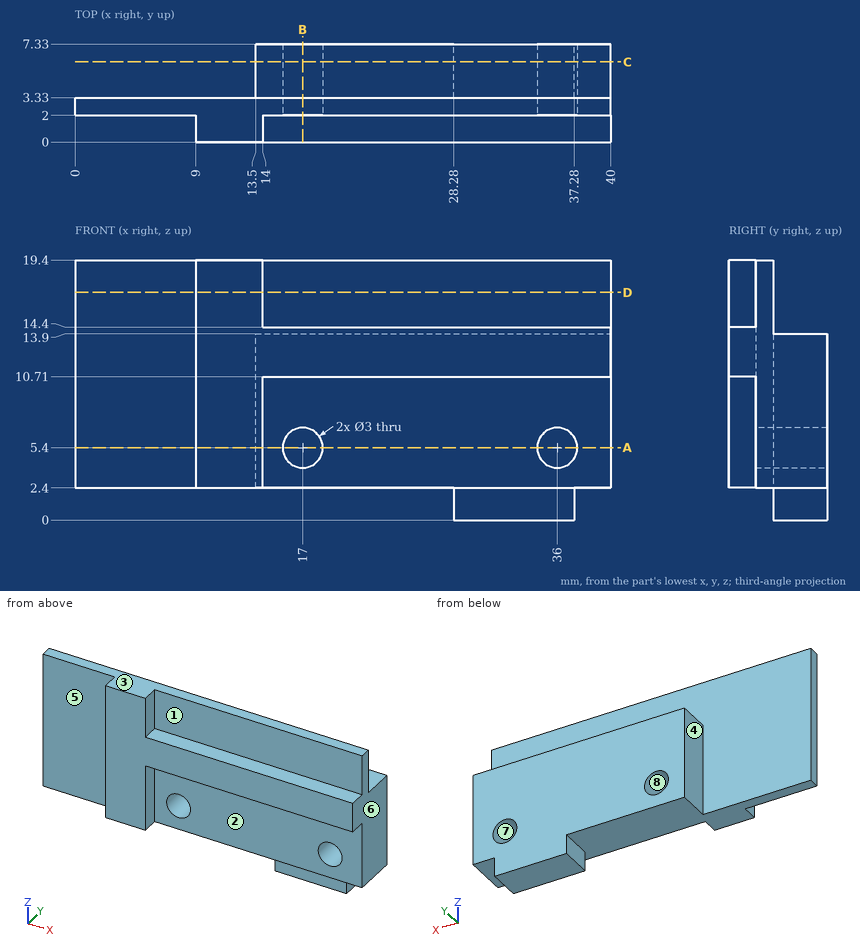
The figure shows three views and two pictorial views of one solid part (mm, origin at its lowest corner). Answer the questions. A direction names the side the tool comes from. Round coordinates to 2 decimals unless told otherwise and drop trailing zeros. Loops run counter-clockwise (first coordinate to the right, second up) from the corner with the lowest first, then second, coordinate; pieces in that order, holes last. Notation, with made-up numbers: (-32, 27) -> (-7, 27) arc R32 ccw to (-7, 66) -> close; hole circle Ø10 at (50.5, 82). An arc over 180 degrees is marked (long way). Use one line per item in the form item = value.
(1) Find section D-D on z = 17. Give the vertices of the cut face in (x, y).
Answer list:
outline = (0, 2) -> (9, 2) -> (9, 0) -> (14, 0) -> (14, 2) -> (40, 2) -> (40, 3.33) -> (0, 3.33) -> close
(2) A tool of negligible diameter and unlimited length cuts with its end or side. For the marked faces 1, 2, 3 and 4, from which of +Z, -Z, +X, -X, +Y, -Y can it reach the whole face along a straight path? Write none if from no direction.
Answer list:
face_1 = +Z, +X, -Y
face_2 = -Z, +X, -Y
face_3 = +Z, +X, -X, +Y, -Y
face_4 = +Z, -Z, -X, +Y
(3) Flat-ended cylindrical pins translate along their axes: P1, Ø4, axis at x = 27.5, z = 8, coming from the -Y side; P2, Ø1.2, axis at y = 4.5, z = 1, coming from the -X side; P3, Ø3, axis at y = 5, z = 9, coming from the -X side; P4, Ø2, axis at y = 1.5, z = 10, coming from the +X side. Find the tip coordinate at first contact, or state that the pin passes through.
Answer list:
P1 = 2
P2 = 28.28
P3 = 13.5
P4 = 40
(4) For a pull along X with two mould halves and no side action, classify the marked faces 5, 6, 7 and 8 as released by +X, released by -X, zero draft, split by the parting line, or undercut.
Answer list:
face_5 = zero draft
face_6 = released by +X
face_7 = undercut
face_8 = undercut
(5) Straight lines are drawn through the part: line 1 (X direction, y = 4.65, z = 5.4); line 2 (X direction, y = 3.1, z = 5.4); line 3 (X direction, y = 0.75, z = 3). For each, find the intervals that lie inside material, in ascending order.
Answer list:
line_1 = 13.5 to 15.5, 18.5 to 34.5, 37.5 to 40
line_2 = 0 to 15.5, 18.5 to 34.5, 37.5 to 40
line_3 = 9 to 14
(6) Find section B-B on x = 17. Give the vertices of the cut face in (y, z), then the cut area to 3 significant figures.
Answer list:
outline = (0, 10.71) -> (2, 10.71) -> (2, 6.9) -> (7.33, 6.9) -> (7.33, 13.9) -> (3.33, 13.9) -> (3.33, 19.4) -> (2, 19.4) -> (2, 14.4) -> (0, 14.4) -> close; (2, 2.4) -> (7.33, 2.4) -> (7.33, 3.9) -> (2, 3.9) -> close
area = 60.0 mm2
(7) Find section C-C on y = 6. Give the vertices of the cut face in (x, z).
Answer list:
outline = (13.5, 2.4) -> (28.28, 2.4) -> (28.28, 0) -> (37.28, 0) -> (37.28, 2.4) -> (40, 2.4) -> (40, 13.9) -> (13.5, 13.9) -> close; hole circle Ø3 at (17, 5.4); hole circle Ø3 at (36, 5.4)
(8) Find section A-A on z = 5.4. Give the vertices of the cut face in (x, y).
Answer list:
outline = (0, 2) -> (9, 2) -> (9, 0) -> (14, 0) -> (14, 2) -> (15.5, 2) -> (15.5, 7.33) -> (13.5, 7.33) -> (13.5, 3.33) -> (0, 3.33) -> close; (18.5, 2) -> (34.5, 2) -> (34.5, 7.33) -> (18.5, 7.33) -> close; (37.5, 2) -> (40, 2) -> (40, 7.33) -> (37.5, 7.33) -> close
